The model under review builds one solid part; all positions refer to its coordinate system, in mm. Round coordinates to 2 decimals unless told otherwise and drop trailing zeros. Order: outer loops, then holes, each group sorted by start corner. A loop starts at its lowest first (then second) coordinate and runs counter-clockwise, first axis right, second up.
1) Consider section D-D (z = -902). Give the boundary of the cut face in (x, y), then the cut area to 3 significant figures.
2) Mouldability with a two-part tool opening along Z and no side actions: class faces 1 (the face through (-84.831, 354.966, -903.788)), 2 (the face through (-85, 332.524, -911)), 3 (the face through (-84.83, 345.26, -895.9)) as pulls with the +Z half, pulls with the -Z half, needs draft (parallel to the pull), parting line crosses it, or undercut.
3) Consider section B-B (x = -84.75). Give the boundary of the cut face in (y, z), then the cut area to 3 significant figures.
4) Clearance check with flat-ended pins moving along their axes: P1, Ø2, axis at x = -86, y = 346.5, coming from the +Z side; P2, Ø2, axis at x = -87, y = 352, coming from the -Z side; P3, Ø6, axis at y = 362.5, z = -916.5, coming from the +X side; P4, Ø6.5, axis at y = 357.22, z = -907.33, coming from the +X side. State where each tip first meets the part, or that it passes through.
5) To check wall thickness, follow L1, parallel to Y at x = -85.5, z = -911; L2, parallel to Z at x = -84.25, y = 357.5; L3, parallel to Z at x = -82.25, y = 360. State the ranges of each line that lie inside material, in increasing order.
6) Consider section A-A (z = -908). Give the boundary of the cut face in (x, y), then the cut area to 3 significant figures.
7) Consider section C-C (y = 340.5). Give the boundary of the cut face in (x, z).
from build123d import *

# Parameters (mm, degrees)
SKETCH1_R           = 4.2
BOSS_EXTRUDE1_DEPTH = 6.35


with BuildPart() as part:
    # Sketch1 → Boss-Extrude1 (new body)
    with BuildSketch(Plane.ZY.offset(81.7)):
        with BuildLine():
            Line((-916.713582015, 360.677443288), (-927.075106991, 332.523601629))
            Line((-927.075106991, 332.523601629), (-894.448362552, 332.523601629))
            Line((-894.448362552, 332.523601629), (-897.39332308, 358.356278755))
            ThreePointArc((-897.39332308, 358.356278755), (-906.13613116, 367.152203744), (-916.713582015, 360.677443288))
        make_face()
        with Locations(Location((-907.328968128, 357.223601629, 0), (0, 0, 270))):
            Circle(SKETCH1_R, mode=Mode.SUBTRACT)
    extrude(amount=BOSS_EXTRUDE1_DEPTH)


solid = part.part
Answer below:
1. outline: (-88.05, 332.52) - (-81.7, 332.52) - (-81.7, 365.69) - (-88.05, 365.69) - close
1. area: 211 mm2
2. face 1: undercut
2. face 2: needs draft
2. face 3: pulls with the +Z half
3. outline: (332.52, -927.08) - (360.68, -916.71) arc R10 ccw to (358.36, -897.39) - (332.52, -894.45) - close; hole circle Ø8.4 at (357.22, -907.33)
3. area: 761 mm2
4. P1: stops at z = -895.93
4. P2: stops at z = -920.28
4. P3: stops at x = -81.7
4. P4: passes through
5. L1: y = 332.52 to 355.18, 359.26 to 366.53
5. L2: z = -917.88 to -911.52, -903.14 to -897.3
5. L3: z = -916.96 to -910.48, -904.18 to -897.72
6. outline: (-88.05, 332.52) - (-81.7, 332.52) - (-81.7, 353.08) - (-88.05, 353.08) - close; (-88.05, 361.37) - (-81.7, 361.37) - (-81.7, 367.2) - (-88.05, 367.2) - close
6. area: 168 mm2
7. outline: (-88.05, -924.14) - (-81.7, -924.14) - (-81.7, -895.36) - (-88.05, -895.36) - close
